Study the drawing (mm; zero at the part's minimum x, y, z) and answer. Give positions to 0.01 mm unless a question says otherwise; leave off trailing zeros. Write each loop counter-clockwise with the first axis right and the second up, starting at its lowest first coordinate (ties: lowest second). Pieces come first, ordered by that corner, then holes. Notation, with made-up numbers: M 62,58.5 L 71,58.5 A28 ccw 71,94.5 Z; hole C -38.75,57 d6. An arc over 180 degrees is marked long. Use a Markdown table: item, result. Add a question column.
Item 1: A cutting plane is placed at A-A on y = 3.5. Determine the outline of the cut face in (x, z), then the cut area to 3 significant figures.
Item 2: A cutting plane is placed at B-B on x = 5. Determine the outline of the cut face in (y, z).
Item 3: A cutting plane is placed at C-C on z = 0.5. Determine the outline of the cut face in (x, y), then the cut area to 4 significant figures.
Item 4: Consider probe 1 along X at (y, z) = (1.75, 0.25); probe 2 along Y at (x, z) = (5, 0.55); probe 3 along X at (y, z) = (16, 0.4). Determine where each line is inside the solid, lowest interval first. Write a range as [from, to].
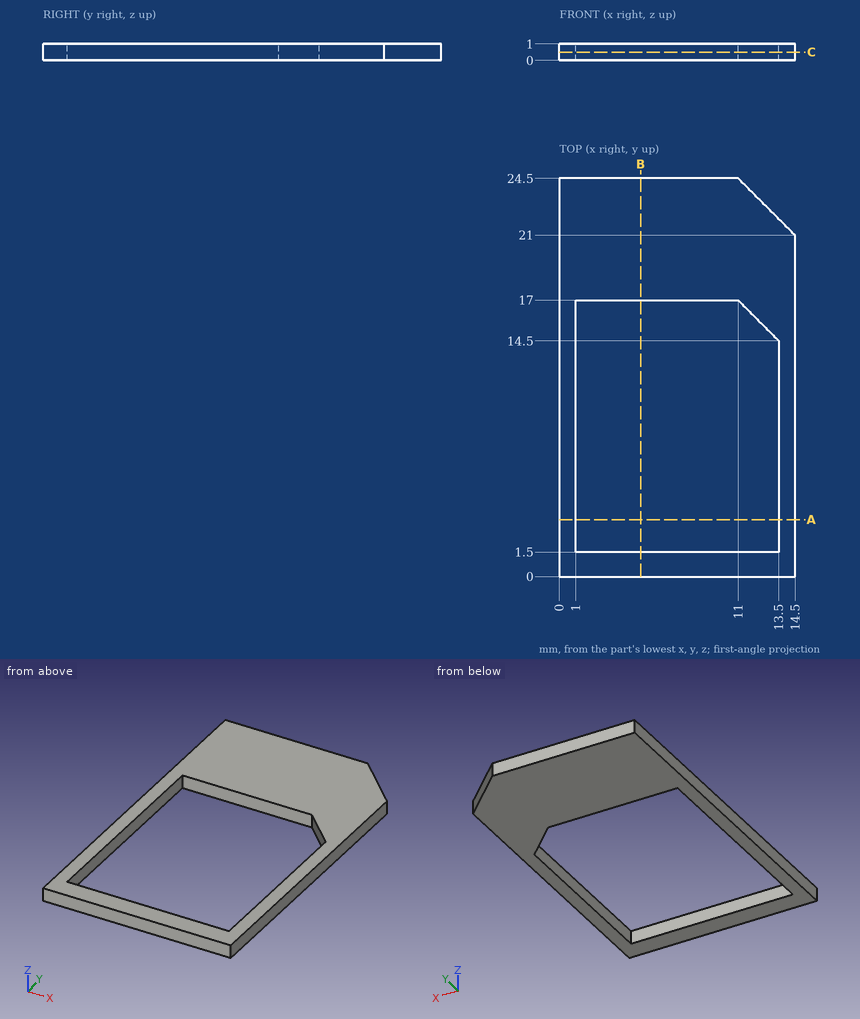
Filled in:
| question | item | result |
|---|---|---|
| 1 | outline | M 0,0 L 1,0 L 1,1 L 0,1 Z; M 13.5,0 L 14.5,0 L 14.5,1 L 13.5,1 Z |
| 1 | area | 2.00 mm² |
| 2 | outline | M 0,0 L 1.5,0 L 1.5,1 L 0,1 Z; M 17,0 L 24.5,0 L 24.5,1 L 17,1 Z |
| 3 | outline | M 0,0 L 14.5,0 L 14.5,21 L 11,24.5 L 0,24.5 Z; hole M 1,1.5 L 13.5,1.5 L 13.5,14.5 L 11,17 L 1,17 Z |
| 3 | area | 158.5 mm² |
| 4 | probe 1 | [0, 1], [13.5, 14.5] |
| 4 | probe 2 | [0, 1.5], [17, 24.5] |
| 4 | probe 3 | [0, 1], [12, 14.5] |
